The model under review builds one solid part; all positions refer to its coordinate system, in mm. Face numbers are marked on the shaded views. Round coordinates to 2 decimals unless told otherwise and drop trailing zeros. Write each loop counter-clockwise with the first axis right and the second up, starting at its lowest first coordinate (ties: lowest second). Pieces come first, ordered by that corner, then holes. Notation, with made-up numbers: (31.25, 35) - (40.25, 35) arc R23 cw to (40.25, 72) - close; hole circle Ø8 at (39.5, 67). An arc over 180 degrees is marked (long way). Write each question's results on one line, items separated by ' | '.
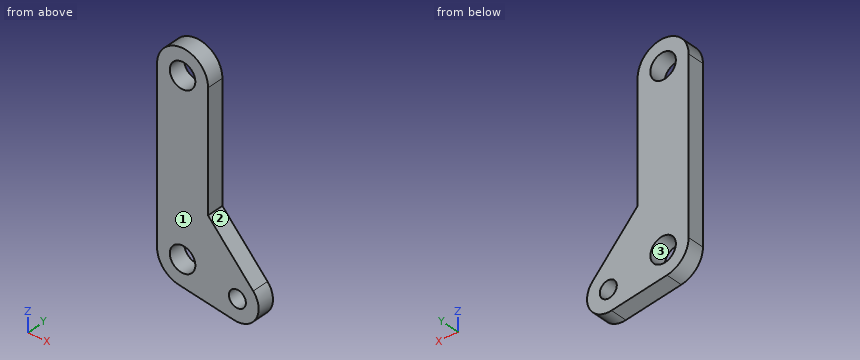
```python
from build123d import *

# Parameters (mm, degrees)
SKETCH1_R           = 1.5
BOSS_EXTRUDE1_DEPTH = 2
BOSS_EXTRUDE2_START = -2
SKETCH2_R           = 1
BOSS_EXTRUDE2_DEPTH = 2


with BuildPart() as part:
    # Sketch1 → Boss-Extrude1 (new body)
    with BuildSketch(Plane(origin=(0, 0, 0), x_dir=(1, 0, 0), z_dir=(0, 1, 0))):
        with BuildLine():
            Line((3, 0), (3, 20))
            ThreePointArc((3, 20), (0, 23), (-3, 20))
            Line((-3, 20), (-3, 0))
            ThreePointArc((-3, 0), (0, -3), (3, 0))
        make_face()
        with Locations(Location((0, 0, 0), (0, 0, 270))):
            Circle(SKETCH1_R, mode=Mode.SUBTRACT)
        with Locations(Location((0, 20, 0), (0, 0, 270))):
            Circle(SKETCH1_R, mode=Mode.SUBTRACT)
    extrude(amount=BOSS_EXTRUDE1_DEPTH)

    # Sketch2 → Boss-Extrude2 (add)
    with BuildSketch(Plane(origin=(0, 2, 0), x_dir=(1, 0, 0), z_dir=(0, 1, 0)).offset(BOSS_EXTRUDE2_START)):
        with BuildLine():
            Line((8.303850429, 19.807351686), (3, 13.914475038))
            Line((3, 13.914475038), (3, 20))
            ThreePointArc((3, 20), (1.956412946, 22.274301735), (-0.448298923, 22.966315573))
            Line((-0.448298923, 22.966315573), (6.072073621, 23.951738706))
            ThreePointArc((6.072073621, 23.951738706), (8.646793057, 22.665134295), (8.303850429, 19.807351686))
        make_face()
        with Locations(Location((6.445656057, 21.479809062, 0), (0, 0, 270))):
            Circle(SKETCH2_R, mode=Mode.SUBTRACT)
    extrude(amount=BOSS_EXTRUDE2_DEPTH)


solid = part.part
```
Q1. Insertion check: P1, Ø2, axis at x = 2.5, z = -5.5, coming from the -Y side. The pin has a flat end and moves straight along its axis. Give the tip position at first contact, or say it passes through.
Evaluation:
P1: stops at y = 0
Q2. We need section D-D (z = -19.5). State the section outline as (x, y) points.
Evaluation:
outline: (-3, 0) - (-1.41, 0) - (-1.41, 2) - (-3, 2) - close; (1.41, 0) - (8.03, 0) - (8.03, 2) - (1.41, 2) - close
Q3. We need section C-C (y = 0.4). State the section outline as (x, z) points.
Evaluation:
outline: (-3, -20) arc R3 ccw to (-0.45, -22.97) - (6.07, -23.95) arc R2.5 ccw to (8.3, -19.81) - (3, -13.91) - (3, 0) arc R3 ccw to (-3, 0) - close; hole circle Ø3 at (0, -20); hole circle Ø3 at (0, 0); hole circle Ø2 at (6.45, -21.48)
Q4. The part is to be moulded in two halves that separate along X. For the marked faces 1, 2 and 3, say which applies: released by +X, released by -X, zero draft, split by the parting line, or undercut.
Evaluation:
face 1: zero draft | face 2: released by +X | face 3: undercut
Q5. We need section A-A (x = 0). State the section outline as (y, z) points, plus the area to 3 significant figures.
Evaluation:
outline: (0, -23.03) - (2, -23.03) - (2, -21.5) - (0, -21.5) - close; (0, -18.5) - (2, -18.5) - (2, -1.5) - (0, -1.5) - close; (0, 1.5) - (2, 1.5) - (2, 3) - (0, 3) - close | area: 40.1 mm^2
Q6. For probe 1 along X at (y, z) = (0.6, 0); probe 2 along Z at (x, y) = (0.25, 0.7); probe 3 along X at (y, z) = (1.45, -10.5), list the stretches that pass through material, from the lowest coordinate up.
Evaluation:
probe 1: x = -3 to -1.5, 1.5 to 3 | probe 2: z = -23.07 to -21.48, -18.52 to -1.48, 1.48 to 2.99 | probe 3: x = -3 to 3
Q7. We need section B-B (z = -0.5). State the section outline as (x, y) points.
Evaluation:
outline: (-3, 0) - (-1.41, 0) - (-1.41, 2) - (-3, 2) - close; (1.41, 0) - (3, 0) - (3, 2) - (1.41, 2) - close
